```python
from build123d import *

# Parameters (mm, degrees)
SKETCH1_R           = 1.45
BOSS_EXTRUDE1_DEPTH = 12
SKETCH2_R           = 2.675
BOSS_EXTRUDE2_DEPTH = 3
CUT_EXTRUDE1_DEPTH  = 2


with BuildPart() as part:
    # Sketch1 → Boss-Extrude1 (new body)
    with BuildSketch(Plane(origin=(0, 0, 0), x_dir=(1, 0, 0), z_dir=(0, 1, 0))):
        with Locations(Location((0, 0, 0), (0, 0, 270))):
            Circle(SKETCH1_R)
    extrude(amount=BOSS_EXTRUDE1_DEPTH)

    # Sketch2 → Boss-Extrude2 (add)
    with BuildSketch(Plane.XZ):
        with Locations(Location((0, 0, 0), (0, 0, 270))):
            Circle(SKETCH2_R)
    extrude(amount=BOSS_EXTRUDE2_DEPTH)

    # Sketch3 → Cut-Extrude1 (cut)
    with BuildSketch(Plane.XZ.offset(3)):
        Polygon((1.661945535, 0.487787902), (0.408536053, 1.683181004), (-1.253409482, 1.195393102), (-1.661945535, -0.487787902), (-0.408536053, -1.683181004), (1.253409482, -1.195393102), align=None)
    extrude(amount=-CUT_EXTRUDE1_DEPTH, mode=Mode.SUBTRACT)


solid = part.part
```
Input: part model. Units: mm. Frame: model coordinates. A direction names the side the tool comes from. Round coordinates to 2 decimals unless told otherwise and drop trailing zeros. Loops run counter-clockwise (first coordinate to the right, second up) from the corner with the lowest first, then second, coordinate; pieces in that order, holes last. Notation, with made-up numbers: M -8.5,-32 L 23.5,-32 A27 cw 23.5,7 Z; hole C 21,-31 d8. An arc over 180 degrees is marked long. Answer in a Markdown table with one row per item. Add a question column.
1. Set-up query: faces 4 (the face through (-0.411, -2.014, 1.443)), 5 (the face through (-1.2, 0, -1.2)), 6 (the face through (-1.2, -3, -1.2)). Return all of +Z, -Z, +X, -X, +Y, -Y with unobstructed straight access to the full face (end or side cutting, diameter ignored); none if empty.
2. Section D-D (y = 0.5). Output: boundary loops of the cut face in (x, z), and give its area (3 significant figures).
3. Contact query for flat-ended pins moving along their axis: pin 1 (2 mm diameter, centred on y = 5, z = 1.5, fed in from +X); pin 2 (3 mm diameter, centred on y = 10.5, z = 1.5, fed in from -X); pin 3 (1.7 mm diameter, centred on x = -0.5, z = 1, fed in from -Y); pin 4 (1 mm diameter, centred on x = 1, y = 2.5, fed in from -Z). Output: stop coordinate, or through.
4. Section A-A (y = -1.5). Output: boundary loops of the cut face in (x, z) (3 decimals), and give its area (3 significant figures).
5. Section B-B (x = 0). Output: boundary loops of the cut face in (y, z) (3 decimals).
6. Section C-C (z = -0.65). Output: boundary loops of the cut face in (x, y).
7. Ray query, probe 1 along Y at (x, z) = (0.35, -0.2); probe 2 along Y at (x, z) = (1.6, 2.1); probe 3 along X at (y, z) = (3.75, -0.05). Return the intervals inside material, ascending.
8. Mould query, pull axis Z, two halves, no side actions, for faces 1 (the face through (0, 12, 0)), 2 (the face through (1.455, -2.014, -0.366)), 3 (the face through (-2.61, -1.48, 0.58)). Classes: released by +Z, released by -Z, zero draft, split by the parting line, or undercut.
Values follow:
| question | item | result |
|---|---|---|
| 1 | face 4 | -Y |
| 1 | face 5 | +Y |
| 1 | face 6 | +Z, -Z, +X, -X, -Y |
| 2 | outline | C 0,0 d2.9 |
| 2 | area | 6.61 mm^2 |
| 3 | pin 1 | x = 1.36 |
| 3 | pin 2 | x = -1.45 |
| 3 | pin 3 | y = -3 |
| 3 | pin 4 | z = -1.36 |
| 4 | outline | C 0,0 d5.35; hole M -1.662,-0.488 L -0.409,-1.683 L 1.253,-1.195 L 1.662,0.488 L 0.409,1.683 L -1.253,1.195 Z |
| 4 | area | 14.7 mm^2 |
| 5 | outline | M -3,-2.675 L 0,-2.675 L 0,-1.45 L 12,-1.45 L 12,1.45 L 0,1.45 L 0,2.675 L -3,2.675 L -3,1.563 L -1,1.563 L -1,-1.563 L -3,-1.563 Z |
| 6 | outline | M -2.59,-3 L -1.49,-3 L -1.49,-1 L 1.39,-1 L 1.39,-3 L 2.59,-3 L 2.59,0 L 1.3,0 L 1.3,12 L -1.3,12 L -1.3,0 L -2.59,0 Z |
| 7 | probe 1 | -1 to 12 |
| 7 | probe 2 | -3 to 0 |
| 7 | probe 3 | -1.45 to 1.45 |
| 8 | face 1 | zero draft |
| 8 | face 2 | undercut |
| 8 | face 3 | split by the parting line |
